```python
from build123d import *

# Parameters (mm, degrees)
BOSS_EXTRUDE1_DEPTH = 40
SKETCH3_R           = 10
SKETCH3_R_2         = 1
CUT_EXTRUDE1_DEPTH  = 3
SKETCH8_R           = 10
BOSS_EXTRUDE2_DEPTH = 15
SKETCH9_W           = 100
SKETCH9_H           = 75
BOSS_EXTRUDE3_DEPTH = 20
FILLET2_R           = 5
FILLET3_R           = 5


with BuildPart() as part:
    # Sketch2 → Boss-Extrude1 (new body)
    with BuildSketch(Plane(origin=(0, 0, 0), x_dir=(1, 0, 0), z_dir=(0, 1, 0))):
        Polygon((-107.5, -15.741355231), (107.5, -15.741355231), (142.5, -80.741355231), (-142.5, -80.741355231), align=None)
    extrude(amount=BOSS_EXTRUDE1_DEPTH)

    # Sketch3 → Cut-Extrude1 (cut)
    with BuildSketch(Plane.XY.offset(80.741355231)):
        with Locations((-64.5, 20)):
            Circle(SKETCH3_R)
        with Locations((-38.5, 20)):
            Circle(SKETCH3_R_2)
        with Locations((-14.5, 20)):
            Circle(SKETCH3_R)
        with Locations((11.5, 20)):
            Circle(SKETCH3_R)
    extrude(amount=-CUT_EXTRUDE1_DEPTH, mode=Mode.SUBTRACT)

    # Sketch8 → Boss-Extrude2 (add)
    with BuildSketch(Plane.XZ):
        with Locations((0, 48.241355231)):
            Circle(SKETCH8_R)
    extrude(amount=BOSS_EXTRUDE2_DEPTH)

    # Sketch9 → Boss-Extrude3 (add)
    with BuildSketch(Plane.XZ.offset(15)):
        with Locations((0, 48.241355231)):
            Rectangle(SKETCH9_W, SKETCH9_H)
    extrude(amount=BOSS_EXTRUDE3_DEPTH)

    # Fillet2
    fillet2_edges = [part.edges().sort_by_distance(p)[0] for p in [
        (-142.5, 20, 80.741355231),
        (-107.5, 20, 15.741355231),
        (107.5, 20, 15.741355231),
        (142.5, 20, 80.741355231),
    ]]
    fillet(fillet2_edges, radius=FILLET2_R)

    # Fillet3
    fillet3_edges = [part.edges().sort_by_distance(p)[0] for p in [
        (50, -25, 10.741355231),
        (50, -25, 85.741355231),
        (-50, -25, 85.741355231),
        (-50, -25, 10.741355231),
    ]]
    fillet(fillet3_edges, radius=FILLET3_R)


solid = part.part
```
Could you check a few things on this model? Use its own coordinates, in mm. A direction names the side the tool comes from. Round coordinates to 2 decimals unless told otherwise and drop trailing zeros. Write each loop counter-clockwise with the first axis right and the second up, starting at its lowest first coordinate (ties: lowest second). Pieces come first, ordered by that corner, then holes. Notation, with made-up numbers: M 78.25,86.25 L 84.25,86.25 A18 cw 84.25,95.25 Z; hole C 82,-3.75 d3. An arc over 180 degrees is marked long. Answer in a Markdown table with one row per item. Add a question column.
Q1. Imagine slicing it at D-D (z = 54). Please give me the cut outline in (x, y).
Q2. On a 3-axis mill with a long thin cutter (end or side, diameter ignored), from which of +Z, -Z, +X, -X, +Y, -Y can I reach the whole of each face in a straight line? I mean faces 5 (the flat face through (50, -25, 48)), 6 (the flat face through (-1, 20, 15.741)), 7 (the cylindrical face through (-74.49, 20.44, 79.26)). Say none if no direction works.
Q3. Imagine slicing it at B-B (y = 4). Please give me the cut outline in (x, z).
Q4. Imagine slicing it at C-C (x = -64.5). Please give me the cut outline in (y, z), then the cut area to 3 significant figures.
Q5. Will these pins go through, and if not, where does the flat tip stop? pin 1 Ø22 at (y, z) = (-21, 32) entering from -X; pin 2 Ø1.5 at (x, y) = (-17, 1) entering from -Z; pin 3 Ø10 at (x, y) = (-12.5, 17.5) entering from +Z.
Q6. If I drill on line 1 (Y direction, x = 11.5, z = 79.6); line 2 (Y direction, x = -38.5, z = 78.6); line 3 (Y direction, x = -21.5, z = 26.5), over which ranges is the centre line in solid material (lowest first)? Write a range as from..to.
Q7. Imagine slicing it at A-A (x = 34.5). Please give me the cut outline in (y, z), then the cut area to 3 significant figures.
Q8. If we mould it in two halves opening along X, with no side actions, what happens to faces 1 (the flat face through (11, 20, 77.741)), 2 (the flat face through (123.52, 19.72, 45.49)), 3 (the flat face through (-15, 20, 77.741)), 4 (the flat face through (-50, -25, 48))? For each: +X half, -X half, draft (parallel to the pull), parting line (faces both ways), or undercut.
Values:
| question | item | result |
|---|---|---|
| 1 | outline | M -128.1,0 L -8.18,0 L -8.18,-15 L -50,-15 L -50,-35 L 50,-35 L 50,-15 L 8.18,-15 L 8.18,0 L 128.1,0 L 128.1,40 L -128.1,40 Z |
| 2 | face 5 | +Z, -Z, +X, -Y |
| 2 | face 6 | -Z, +X, -X, +Y |
| 2 | face 7 | +Z |
| 3 | outline | M -138.53,73.37 L -108.92,18.37 A5 ccw -104.51,15.74 L 104.51,15.74 A5 ccw 108.92,18.37 L 138.53,73.37 A5 ccw 134.13,80.74 L -134.13,80.74 A5 ccw Z |
| 4 | outline | M 0,15.74 L 40,15.74 L 40,80.74 L 30,80.74 L 30,77.74 L 10,77.74 L 10,80.74 L 0,80.74 Z |
| 4 | area | 2,540 mm^2 |
| 5 | pin 1 | x = -50 |
| 5 | pin 2 | z = 15.74 |
| 5 | pin 3 | z = 77.74 |
| 6 | line 1 | -35..-15, 0..10, 30..40 |
| 6 | line 2 | -35..-15, 0..19, 21..40 |
| 6 | line 3 | -35..-15, 0..40 |
| 7 | outline | M -35,10.74 L -15,10.74 L -15,85.74 L -35,85.74 Z; M 0,15.74 L 40,15.74 L 40,80.74 L 0,80.74 Z |
| 7 | area | 4,100 mm^2 |
| 8 | face 1 | undercut |
| 8 | face 2 | +X half |
| 8 | face 3 | undercut |
| 8 | face 4 | -X half |
